Design review of the part built by this model. Coordinates are the model's own, in mm. A direction names the side the tool comes from. Coordinates: 2 decimals unless noted, no trailing zeros. Loops run counter-clockwise (first coordinate to the right, second up) from the corner with the lowest first, then second, coordinate; pieces in that order, holes last. Notation, with made-up numbers: M 26.5,18.5 L 84.5,18.5 A9 ccw 84.5,32.5 Z; hole C 38,15.25 d6. An arc over 180 degrees is marked long. Write item = value, one per line. Start each with the question number.
```python
from build123d import *

# Parameters (mm, degrees)
SKETCH1_R           = 4.35
SKETCH1_R_2         = 4.99
BOSS_EXTRUDE1_DEPTH = 5
FILLET1_R           = 15
FILLET2_R           = 20
FILLET3_R           = 20
CUT_EXTRUDE1_DEPTH  = 109.301776601
FILLET4_R           = 5
FILLET5_R           = 3
FILLET6_R           = 3


with BuildPart() as part:
    # Sketch1 → Boss-Extrude1 (new body)
    with BuildSketch(Plane.XY):
        Polygon((0, 91.64845728), (0, 0), (114.5605716, 0), align=None)
        with Locations((16.765578361, 56.765578361)):
            Circle(SKETCH1_R, mode=Mode.SUBTRACT)
        with Locations((66.765578361, 16.765578361)):
            Circle(SKETCH1_R, mode=Mode.SUBTRACT)
        with Locations((16.765578361, 16.765578361)):
            Circle(SKETCH1_R_2, mode=Mode.SUBTRACT)
    extrude(amount=BOSS_EXTRUDE1_DEPTH)

    # Fillet1
    fillet1_edges = [part.edges().sort_by_distance(p)[0] for p in [
        (0, 91.64845728, 2.5),
    ]]
    fillet(fillet1_edges, radius=FILLET1_R)

    # Fillet2
    fillet2_edges = [part.edges().sort_by_distance(p)[0] for p in [
        (0, 0, 2.5),
    ]]
    fillet(fillet2_edges, radius=FILLET2_R)

    # Fillet3
    fillet3_edges = [part.edges().sort_by_distance(p)[0] for p in [
        (114.5605716, 0, 2.5),
    ]]
    fillet(fillet3_edges, radius=FILLET3_R)

    # Sketch2 → Cut-Extrude1 (cut, through all)
    with BuildSketch(Plane.XY.offset(5)):
        Polygon((21.265578361, 47.402766547), (53.937063594, 21.265578361), (21.265578361, 21.265578361), align=None)
    extrude(amount=-CUT_EXTRUDE1_DEPTH, mode=Mode.SUBTRACT)

    # Fillet4
    fillet4_edges = [part.edges().sort_by_distance(p)[0] for p in [
        (21.265578361, 21.265578361, 2.5),
    ]]
    fillet(fillet4_edges, radius=FILLET4_R)

    # Fillet5
    fillet5_edges = [part.edges().sort_by_distance(p)[0] for p in [
        (21.265578361, 47.402766547, 2.5),
    ]]
    fillet(fillet5_edges, radius=FILLET5_R)

    # Fillet6
    fillet6_edges = [part.edges().sort_by_distance(p)[0] for p in [
        (53.937063594, 21.265578361, 2.5),
    ]]
    fillet(fillet6_edges, radius=FILLET6_R)


solid = part.part
```
(1) Tool access review of faces 4 (the flat face through (21.266, 34, 3)), 5 (the cylindrical face through (8.29, 73.855, 2.535)): name each direction out of +Z, -Z, +X, -X, +Y, -Y from which nothing blocks a thin tool from reaching the whole face with its end or side.
(2) Mouldability with a two-part tool opening along X and no side actions: class faces 1 (the cylindrical face through (76.3, 13.05, 2.54)), 2 (the cylindrical face through (22.69, 22.77, 2.46)), 3 (the flat face through (0, 41, 2)) as +X half, -X half, draft (parallel to the pull), parting line (faces both ways), or undercut.
(3) To check wall thickness, follow L1, parallel to X at y = 17, z = 2.4; L2, parallel to X at y = 20.5, z = 2.75; L3, parallel to Y at x = 18.5, z = 3.9. State the ranges of each line that lie inside material, in increasing order.
(4) Insertion check: pin 1 (2 mm diameter, centred on x = 19.5, z = 3.5, fed in from -Y); pin 2 (1 mm diameter, centred on x = 68, z = 1, fed in from +Y); pin 3 (2 mm diameter, centred on x = 47, z = 1.5, fed in from +Y). Each pin has a flat end and moves straight along its axis. Give the tip position at first contact, or say it passes through.
(5) Take a section at A-A (y = 40). State the section outline as (x, z) points, plus the area to 3 significant figures.
(6) Take a section at D-D (z = 1.9). State the section outline as (x, y) points.
(7) Take a section at B-B (x = 14.5). State the section outline as (y, z) points, plus the area to 3 significant figures.
(8) Take a section at C-C (x = 64). State the section outline as (y, z) points, plus the area to 3 significant figures.
Results list:
q1.face_4 = +Z, -Z
q1.face_5 = +Z, -Z, +Y
q2.face_1 = +X half
q2.face_2 = undercut
q2.face_3 = -X half
q3.L1 = 0.23 to 11.78, 21.75 to 62.42, 71.11 to 77.32
q3.L2 = 0 to 13.46, 20.08 to 64.53, 69 to 77.54
q3.L3 = 0.06 to 12.09, 21.44 to 52.78, 60.75 to 75.03
q4.pin_1 = 0
q4.pin_2 = 37.65
q4.pin_3 = 54.85
q5.outline = M 0,0 L 21.27,0 L 21.27,5 L 0,5 Z; M 30.52,0 L 64.56,0 L 64.56,5 L 30.52,5 Z
q5.area = 277 mm^2
q6.outline = M 0,20 A20 ccw 20,0 L 57.54,0 A20 ccw 70.04,35.62 L 24.37,72.15 A15 ccw 0,60.44 Z; hole C 16.77,16.77 d9.98; hole C 16.77,56.77 d8.7; hole M 21.27,26.27 A5 ccw 26.27,21.27 L 45.38,21.27 A3 ccw 47.26,26.61 L 26.14,43.5 A3 ccw 21.27,41.16 Z; hole C 66.77,16.77 d8.7
q7.outline = M 0.77,0 L 12.32,0 L 12.32,5 L 0.77,5 Z; M 21.21,0 L 53.05,0 L 53.05,5 L 21.21,5 Z; M 60.48,0 L 75.43,0 L 75.43,5 L 60.48,5 Z
q7.area = 292 mm^2
q8.outline = M 1.07,0 L 13.41,0 L 13.41,5 L 1.07,5 Z; M 20.12,0 L 40.45,0 L 40.45,5 L 20.12,5 Z
q8.area = 163 mm^2
